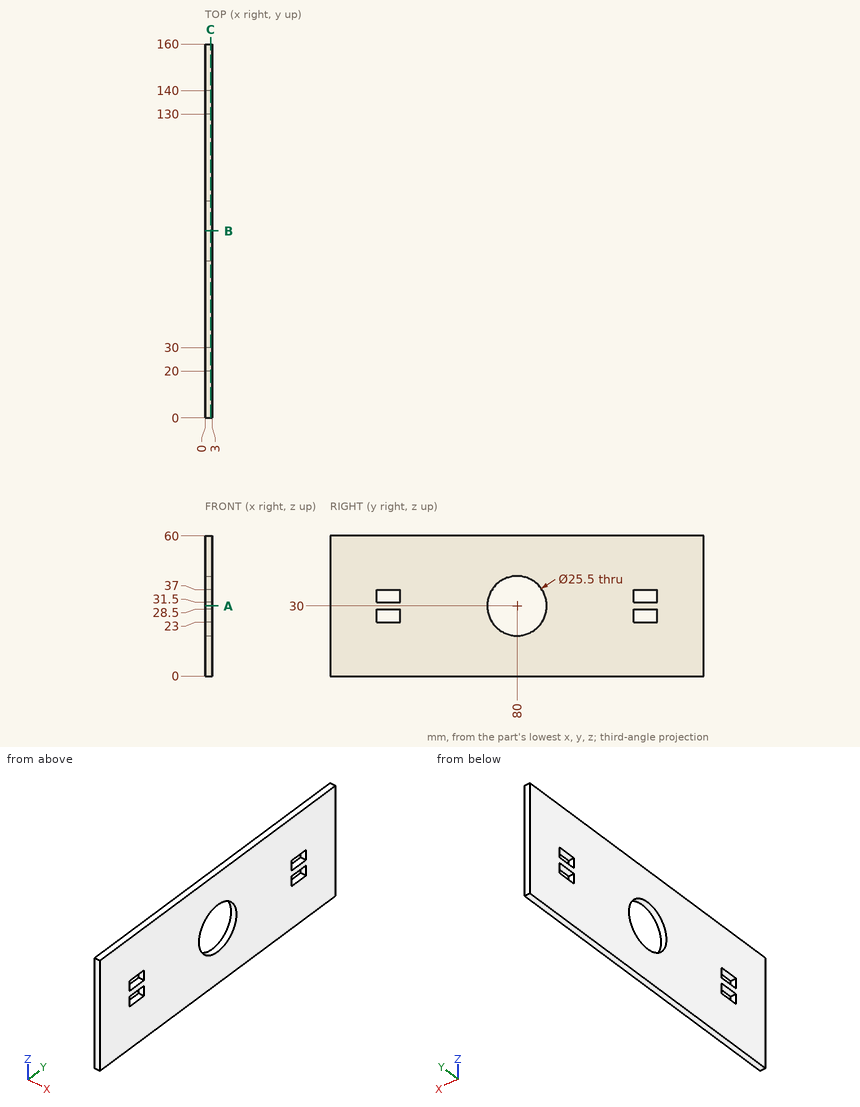
Design review of the part shown in the three views and the two pictorial views. Dimensions are in mm from the part's minimum x, y and z. Round coordinates to 2 decimals unless told otherwise and drop trailing zeros. Loops run counter-clockwise (first coordinate to the right, second up) from the corner with the lowest first, then second, coordinate; pieces in that order, holes last. Notation, with made-up numbers: (79.25, 30.25) -> (110.25, 30.25) arc R16 ccw to (110.25, 61.25) -> close; hole circle Ø9 at (69, 19). An arc over 180 degrees is marked (long way). Return JSON: item names as keys, results as strings.
(1) Add section A-A on z = 30. Write out the cut boundary in (x, y).
Solved:
{"outline": "(0, 0) -> (3, 0) -> (3, 67.25) -> (0, 67.25) -> close; (0, 92.75) -> (3, 92.75) -> (3, 160) -> (0, 160) -> close"}
(2) Add section B-B on y = 80. Write out the cut boundary in (x, z).
Solved:
{"outline": "(0, 0) -> (3, 0) -> (3, 17.25) -> (0, 17.25) -> close; (0, 42.75) -> (3, 42.75) -> (3, 60) -> (0, 60) -> close"}
(3) For line 1 (Z direction, x = 2.75, y = 25.5); line 2 (Y direction, x = 1.15, z = 24); line 3 (Z direction, x = 2.25, y = 80), list the stretches that pass through material, from the lowest coordinate up.
Solved:
{"line 1": "0 to 23, 28.5 to 31.5, 37 to 60", "line 2": "0 to 20, 30 to 68.75, 91.25 to 130, 140 to 160", "line 3": "0 to 17.25, 42.75 to 60"}
(4) Add section C-C on x = 2.4. Write out the cut boundary in (y, z).
Solved:
{"outline": "(0, 0) -> (160, 0) -> (160, 60) -> (0, 60) -> close; hole (20, 23) -> (30, 23) -> (30, 28.5) -> (20, 28.5) -> close; hole (20, 31.5) -> (30, 31.5) -> (30, 37) -> (20, 37) -> close; hole circle Ø25.5 at (80, 30); hole (130, 23) -> (140, 23) -> (140, 28.5) -> (130, 28.5) -> close; hole (130, 31.5) -> (140, 31.5) -> (140, 37) -> (130, 37) -> close"}
